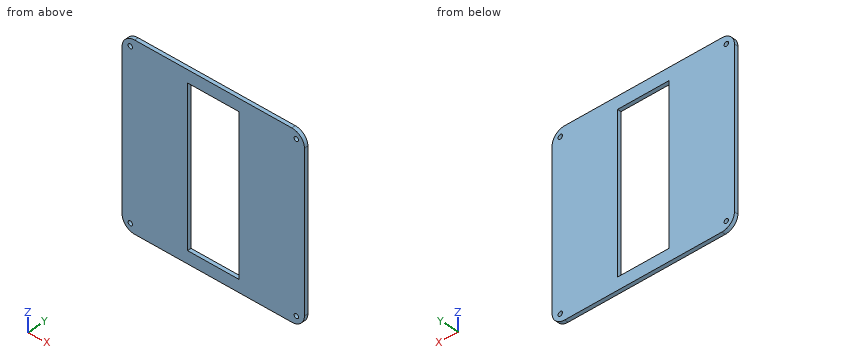
```python
from build123d import *

# Parameters (mm, degrees)
ESQUISSE1_R        = 1.75
ESQUISSE1_W        = 41
ESQUISSE1_H        = 126.2
BOSS_EXTRU_1_DEPTH = 3


with BuildPart() as part:
    # Esquisse1 → Boss.-Extru.1 (new body)
    with BuildSketch(Plane(origin=(0, 0, 0), x_dir=(1, 0, 0), z_dir=(0, 1, 0))):
        with BuildLine():
            Line((-72.6, -63.1), (-72.6, 63.1))
            ThreePointArc((-72.6, 63.1), (-69.671067812, 70.171067812), (-62.6, 73.1))
            Line((-62.6, 73.1), (62.6, 73.1))
            ThreePointArc((62.6, 73.1), (69.671067812, 70.171067812), (72.6, 63.1))
            Line((72.6, 63.1), (72.6, -63.1))
            ThreePointArc((72.6, -63.1), (69.671067812, -70.171067812), (62.6, -73.1))
            Line((62.6, -73.1), (-62.6, -73.1))
            ThreePointArc((-62.6, -73.1), (-69.671067812, -70.171067812), (-72.6, -63.1))
        make_face()
        with Locations(Location((-66.1, 66.6, 0), (0, 0, 270))):
            Circle(ESQUISSE1_R, mode=Mode.SUBTRACT)
        with Locations(Location((66.1, 66.6, 0), (0, 0, 270))):
            Circle(ESQUISSE1_R, mode=Mode.SUBTRACT)
        with Locations(Location((66.1, -66.6, 0), (0, 0, 270))):
            Circle(ESQUISSE1_R, mode=Mode.SUBTRACT)
        with Locations(Location((-66.1, -66.6, 0), (0, 0, 270))):
            Circle(ESQUISSE1_R, mode=Mode.SUBTRACT)
        Rectangle(ESQUISSE1_W, ESQUISSE1_H, mode=Mode.SUBTRACT)
    extrude(amount=BOSS_EXTRU_1_DEPTH)


solid = part.part
```
Geometry: final body of the model. Coordinates: model frame, mm. Coordinates: 2 decimals unless noted, no trailing zeros. Order: outer loops, then holes, each group sorted by start corner. A loop starts at its lowest first (then second) coordinate and runs counter-clockwise, first axis right, second up. Notation, with made-up numbers: (42.25, 52.25) - (85.25, 52.25) arc R30 ccw to (85.25, 81.25) - close; hole circle Ø11 at (19, 79.5). An arc over 180 degrees is marked (long way). Return JSON: item names as keys, results as strings. Group by question number.
1. Material intervals for line 1 along X through (y, z) = (0.95, -45); line 2 along Z through (x, y) = (-20, 2.75); line 3 along X through (y, z) = (2, -66.6), sorted ascending. Write a range as [from, to].
2. Cut plane A-A (z = 9). Output: boundary loops of the cut face in (x, y).
3. Cut plane B-B (x = 8.5). Output: boundary loops of the cut face in (y, z), plus the area to 3 significant figures.
4. Cut plane D-D (x = 66.1). Output: boundary loops of the cut face in (y, z), plus the area to 3 significant figures.
5. Cut plane C-C (y = 0.8). Output: boundary loops of the cut face in (x, z), plus the area to 3 significant figures.
Resolved:
{
 "1": {"line 1": "x = [-72.6, -20.5], [20.5, 72.6]", "line 2": "z = [-73.1, -63.1], [63.1, 73.1]", "line 3": "x = [-71.97, -67.85], [-64.35, 64.35], [67.85, 71.97]"},
 "2": {"outline": "(-72.6, 0) - (-20.5, 0) - (-20.5, 3) - (-72.6, 3) - close; (20.5, 0) - (72.6, 0) - (72.6, 3) - (20.5, 3) - close"},
 "3": {"outline": "(0, -73.1) - (3, -73.1) - (3, -63.1) - (0, -63.1) - close; (0, 63.1) - (3, 63.1) - (3, 73.1) - (0, 73.1) - close", "area": "60.0 mm²"},
 "4": {"outline": "(0, -72.47) - (3, -72.47) - (3, -68.35) - (0, -68.35) - close; (0, -64.85) - (3, -64.85) - (3, 64.85) - (0, 64.85) - close; (0, 68.35) - (3, 68.35) - (3, 72.47) - (0, 72.47) - close", "area": "414 mm²"},
 "5": {"outline": "(-72.6, -63.1) arc R10 ccw to (-62.6, -73.1) - (62.6, -73.1) arc R10 ccw to (72.6, -63.1) - (72.6, 63.1) arc R10 ccw to (62.6, 73.1) - (-62.6, 73.1) arc R10 ccw to (-72.6, 63.1) - close; hole circle Ø3.5 at (-66.1, -66.6); hole circle Ø3.5 at (-66.1, 66.6); hole (-20.5, -63.1) - (20.5, -63.1) - (20.5, 63.1) - (-20.5, 63.1) - close; hole circle Ø3.5 at (66.1, -66.6); hole circle Ø3.5 at (66.1, 66.6)", "area": "15,900 mm²"}
}
